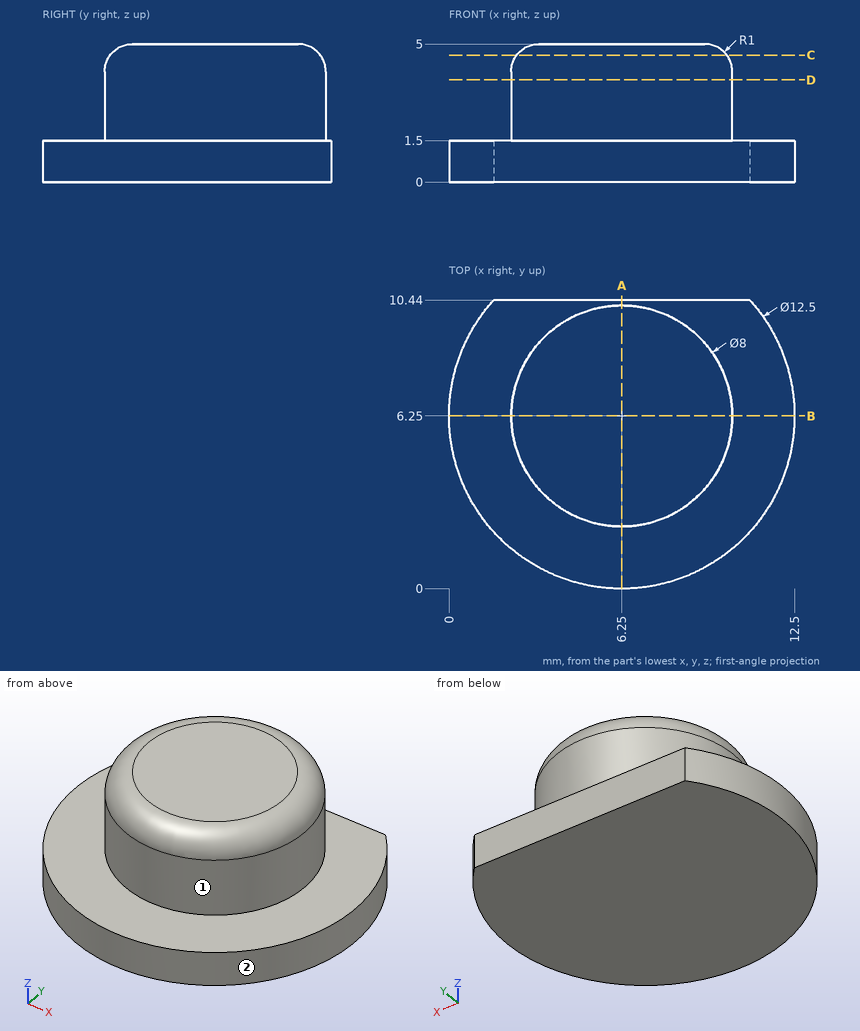
Design review of the part shown in the three views and the two pictorial views. Dimensions are in mm from the part's minimum x, y and z. A direction names the side the tool comes from. Round coordinates to 2 decimals unless told otherwise and drop trailing zeros. Loops run counter-clockwise (first coordinate to the right, second up) from the corner with the lowest first, then second, coordinate; pieces in that order, holes last. Notation, with made-up numbers: (16.5, 68) -> (48.5, 68) arc R33 ccw to (48.5, 96) -> close; hole circle Ø6 at (41, -32.5). An arc over 180 degrees is marked (long way). Use one line per item in the form item = value. Start each with the question number.
Q1. We need section C-C on z = 4.6. Give the boundary of the cut face in (x, y).
Q2. We need section A-A on x = 6.25. Give the boundary of the cut face in (y, z).
Q3. We need section D-D on z = 3.7. Give the boundary of the cut face in (x, y).
Q4. For pin 1 Ø1 at (x, z) = (7, 2.5) entering from +Y; pin 2 Ø6 at (x, y) = (2.5, 7.5) entering from +Z; pin 3 Ø1.5 at (x, y) = (9, 3) entering from +Z; pin 4 Ø1.5 at (y, z) = (6.5, 4) entering from +X, all flat-tipped, find the tip position at first contact; note any pin that passes through.
Q5. We need section B-B on y = 6.25. Give the boundary of the cut face in (x, z).
Q6. Wall thickness on line 1 along Z through (x, y) = (11, 3); line 2 along Z through (x, y) = (7, 9.25); line 3 along Y through (x, z) = (9.75, 0.3): over which ranges is each line inside the solid? List them lowest first. Write a range as [from, to].
Q7. Machinability: for the marked faces 1 and 2, which of the approach directions +Z, -Z, +X, -X, +Y, -Y give a long, thin tool a straight path to every point of the face, cutting with its end or side? Answer none if there is none.
Calculated:
q1.outline = circle Ø7.6 at (6.25, 6.25)
q2.outline = (0, 0) -> (10.44, 0) -> (10.44, 1.5) -> (10.25, 1.5) -> (10.25, 4) arc R1 ccw to (9.25, 5) -> (3.25, 5) arc R1 ccw to (2.25, 4) -> (2.25, 1.5) -> (0, 1.5) -> close
q3.outline = circle Ø8 at (6.25, 6.25)
q4.pin_1 = 10.24
q4.pin_2 = 5
q4.pin_3 = 4.86
q4.pin_4 = 10.25
q5.outline = (0, 0) -> (12.5, 0) -> (12.5, 1.5) -> (10.25, 1.5) -> (10.25, 4) arc R1 ccw to (9.25, 5) -> (3.25, 5) arc R1 ccw to (2.25, 4) -> (2.25, 1.5) -> (0, 1.5) -> close
q6.line_1 = [0, 1.5]
q6.line_2 = [0, 5]
q6.line_3 = [1.07, 10.44]
q7.face_1 = +Z
q7.face_2 = +Z, -Z
